```python
from build123d import *

# Parameters (mm, degrees)
F0_W     = 177.8
F0_H     = 279.4
F0_R     = 38.5
F1_DEPTH = 56.515
F3_DEPTH = 177.801
F5_DEPTH = 177.801
F6_R     = 6.746875
F7_DEPTH = 20.8223992262
F8_R     = 5.5
F9_DEPTH = 113.031


with BuildPart() as f1:
    # F0 (on Front) → F1 (new body, symmetric)
    with BuildSketch(Plane.XZ):
        with Locations((0, -12.7)):
            Rectangle(F0_W, F0_H)
        Circle(F0_R, mode=Mode.SUBTRACT)
    extrude(amount=F1_DEPTH, both=True)

    # F2 (on face) → F3 (cut, through all)
    with BuildSketch(Plane.YZ.offset(88.9)):
        with BuildLine():
            ThreePointArc((22.9936007738, -131.5786007738), (31.9738568949, -127.8588568949), (35.6936007738, -118.8786007738))
            Line((35.6936007738, -118.8786007738), (35.6936007738, 93.4786007738))
            ThreePointArc((35.6936007738, 93.4786007738), (31.9738568949, 102.4588568949), (22.9936007738, 106.1786007738))
            Line((22.9936007738, 106.1786007738), (-22.9936007738, 106.1786007738))
            ThreePointArc((-22.9936007738, 106.1786007738), (-31.9738568949, 102.4588568949), (-35.6936007738, 93.4786007738))
            Line((-35.6936007738, 93.4786007738), (-35.6936007738, -118.8786007738))
            ThreePointArc((-35.6936007738, -118.8786007738), (-31.9738568949, -127.8588568949), (-22.9936007738, -131.5786007738))
            Line((-22.9936007738, -131.5786007738), (22.9936007738, -131.5786007738))
        make_face()
    extrude(amount=-F3_DEPTH, mode=Mode.SUBTRACT)

    # F4 (on face) → F5 (cut, through all)
    with BuildSketch(Plane(origin=(-88.9, 0, 0), x_dir=(0, -1, 0), z_dir=(-1, 0, 0))):
        with BuildLine():
            Line((45.72, 53.975), (-45.72, 53.975))
            ThreePointArc((-45.72, 53.975), (-50.2101280605, 52.1151280605), (-52.07, 47.625))
            Line((-52.07, 47.625), (-52.07, -47.625))
            ThreePointArc((-52.07, -47.625), (-50.2101280605, -52.1151280605), (-45.72, -53.975))
            Line((-45.72, -53.975), (45.72, -53.975))
            ThreePointArc((45.72, -53.975), (50.2101280605, -52.1151280605), (52.07, -47.625))
            Line((52.07, -47.625), (52.07, 47.625))
            ThreePointArc((52.07, 47.625), (50.2101280605, 52.1151280605), (45.72, 53.975))
        make_face()
    extrude(amount=-F5_DEPTH, mode=Mode.SUBTRACT)

    # F6 (on face) → F7 (cut, through all)
    with BuildSketch(Plane.XY.offset(-131.5786007738)):
        with Locations((63.103125, 0)):
            Circle(F6_R)
        with Locations((-63.103125, 0)):
            Circle(F6_R)
    extrude(amount=-F7_DEPTH, mode=Mode.SUBTRACT)

    # F8 (on face) → F9 (cut, through all)
    with BuildSketch(Plane.XZ.offset(56.515)):
        with Locations((49.5, -85.7365149747)):
            Circle(F8_R)
    extrude(amount=-F9_DEPTH, mode=Mode.SUBTRACT)


solid = f1.part
```
Could you check a few things on this model? Use its own coordinates, in mm. A direction names the side the tool comes from. Round coordinates to 2 decimals unless told otherwise and drop trailing zeros. Loops run counter-clockwise (first coordinate to the right, second up) from the corner with the lowest first, then second, coordinate; pieces in that order, holes last.
Q1. Please list where these lines run through material, in increasing order: L1, parallel to Z at x = 0, y = -55.15; L2, parallel to Y at x = 52, z = -112 (3 decimals); L3, parallel to Y at x = 65, z = -29.5 (3 decimals).
Q2. I want a section at D-D (z = -67). Write out the boundary of the cut face in (x, y) (3 decimals).
Q3. I want a section at C-C (y = 0). Write out the boundary of the cut face in (x, z), and give its area (3 significant figures).
Q4. On a 3-axis mill with a long thin cutter (end or side, diameter ignored), from which of +Z, -Z, +X, -X, +Y, -Y can I reach the whole of each face in a straight line? I mean faces 1 (the cylindrical face through (44.005, 45.959, -85.495)), 2 (the flat face through (1, -35.694, 74)), 3 (the cylindrical face through (69.538, 2.027, -141.844)). Say none if no direction works.
Q5. Thinking about a two-plate mould opening in Y: for faces 4 (the cylindrical face through (-30.55, 54.32, -23.43)), 5 (the flat face through (1, 35.694, -87)), 6 (the flat face through (-1, 56.515, -42)), which applies, pulls with the +Y half, pulls with the -Y half, needs draft (parallel to the pull), parting line crosses it, or undercut?
Q6. For P1, Ø12.5, axis at x = 49.5, z = -85.74, coming from the +Y side (3 decimals), with a flat end and sliding along its axis, tell me the tip position at first contact or that it passes through.
Q7. I want a section at B-B (z = 0). Write out the boundary of the cut face in (x, y) (3 decimals).
Answer below:
1. L1: z = -152.4 to -38.5, 38.5 to 127
1. L2: y = -56.515 to -35.694, 35.694 to 56.515
1. L3: y = -56.515 to -52.07, 52.07 to 56.515
2. outline: (-88.9, -56.515) - (88.9, -56.515) - (88.9, -35.694) - (-88.9, -35.694) - close; (-88.9, 35.694) - (88.9, 35.694) - (88.9, 56.515) - (-88.9, 56.515) - close
3. outline: (-88.9, -152.4) - (-69.85, -152.4) - (-69.85, -131.58) - (-88.9, -131.58) - close; (-88.9, 106.18) - (88.9, 106.18) - (88.9, 127) - (-88.9, 127) - close; (-56.36, -152.4) - (56.36, -152.4) - (56.36, -131.58) - (-56.36, -131.58) - close; (69.85, -152.4) - (88.9, -152.4) - (88.9, -131.58) - (69.85, -131.58) - close
3. area: 6,840 mm2
4. face 1: +Y, -Y
4. face 2: +X, -X
4. face 3: -Z
5. face 4: needs draft
5. face 5: undercut
5. face 6: pulls with the +Y half
6. P1: stops at y = 56.515
7. outline: (-88.9, -56.515) - (-38.5, -56.515) - (-38.5, -52.07) - (-88.9, -52.07) - close; (-88.9, 52.07) - (-38.5, 52.07) - (-38.5, 56.515) - (-88.9, 56.515) - close; (38.5, -56.515) - (88.9, -56.515) - (88.9, -52.07) - (38.5, -52.07) - close; (38.5, 52.07) - (88.9, 52.07) - (88.9, 56.515) - (38.5, 56.515) - close
